```python
from build123d import *

# Parameters (mm, degrees)
F0_W                 = 20
F0_H                 = 40
F0_R                 = 3
F0_H_2               = 20
F0_R_2               = 5
F0_W_2               = 40
F1_DEPTH             = 3
F0_W_3               = 3
F0_H_3               = 3
F2_DEPTH             = 23
F3_DEPTH             = 63
F4_R                 = 3
F4_R_2               = 5
F6_DEPTH             = 25
F5_R                 = 3
F5_R_2               = 5
F7_DEPTH             = 25
F8_DEPTH             = 23
F9_D                 = 6
F9_DEPTH             = 23
F9_CBORE_D           = 10
F9_CBORE_DEPTH       = 21
F9_TIP               = 1.8025818571
F9_ON_F5_D           = 6
F9_ON_F5_DEPTH       = 23
F9_ON_F5_CBORE_D     = 10
F9_ON_F5_CBORE_DEPTH = 21
F9_ON_F5_TIP         = 1.8025818571
F9_ON_F4_D           = 6
F9_ON_F4_DEPTH       = 23
F9_ON_F4_CBORE_D     = 10
F9_ON_F4_CBORE_DEPTH = 21
F9_ON_F4_TIP         = 1.8025818571


# Not quite as in the source:
# - a feature of the source that left no trace in its solid (it failed there, or was rolled back) is left out


with BuildPart() as f1:
    # F0 (on Front) → F1 (new body)
    with BuildSketch(Plane.XZ):
        with Locations((-10, 20)):
            Rectangle(F0_W, F0_H)
        with Locations((-10, 7.5)):
            Circle(F0_R, mode=Mode.SUBTRACT)
        with Locations((-10, 32.5)):
            Circle(F0_R, mode=Mode.SUBTRACT)
        with Locations((-10, 50)):
            Rectangle(F0_W, F0_H_2)
        with Locations((-10, 50)):
            Circle(F0_R_2, mode=Mode.SUBTRACT)
        with Locations((20, 50)):
            Rectangle(F0_W_2, F0_H_2)
        with Locations((7.5, 50)):
            Circle(F0_R, mode=Mode.SUBTRACT)
        with Locations((32.5, 50)):
            Circle(F0_R, mode=Mode.SUBTRACT)
    extrude(amount=-F1_DEPTH)

    # F0 (on Front) → F2 (join)
    with BuildSketch(Plane.XZ):
        with Locations((-21.5, 20)):
            Rectangle(F0_W_3, F0_H)
        with Locations((20, 61.5)):
            Rectangle(F0_W_2, F0_H_3)
    extrude(amount=-F2_DEPTH)

    # F0 (on Front) → F3 (join)
    with BuildSketch(Plane.XZ):
        Polygon((-20, 60), (0, 60), (0, 63), (-23, 63), (-23, 60), align=None)
        with Locations((-21.5, 50)):
            Rectangle(F0_W_3, F0_H_2)
    extrude(amount=-F3_DEPTH)

    # F4 (on face) → F6 (cut)
    with BuildSketch(Plane.XY.offset(63)):
        with Locations((-10, 55.5)):
            Circle(F4_R)
        with Locations((-10, 30.5)):
            Circle(F4_R)
        with Locations((-10, 13)):
            Circle(F4_R_2)
        with Locations((7.5, 13)):
            Circle(F4_R)
        with Locations((32.5, 13)):
            Circle(F4_R)
    extrude(amount=-F6_DEPTH, mode=Mode.SUBTRACT)

    # F5 (on face) → F7 (cut)
    with BuildSketch(Plane(origin=(-23, 0, 0), x_dir=(0, -1, 0), z_dir=(-1, 0, 0))):
        with Locations((-55.5, 50)):
            Circle(F5_R)
        with Locations((-30.5, 50)):
            Circle(F5_R)
        with Locations((-13, 50)):
            Circle(F5_R_2)
        with Locations((-13, 7.5)):
            Circle(F5_R)
        with Locations((-13, 32.5)):
            Circle(F5_R)
    extrude(amount=-F7_DEPTH, mode=Mode.SUBTRACT)

    # F0 (on Front) → F8 (join)
    with BuildSketch(Plane.XZ):
        with Locations((-10, 50)):
            Rectangle(F0_W, F0_H_2)
        with Locations((-10, 50)):
            Circle(F0_R_2, mode=Mode.SUBTRACT)
        Polygon((-20, 60), (0, 60), (0, 63), (-23, 63), (-23, 60), align=None)
        with Locations((-21.5, 50)):
            Rectangle(F0_W_3, F0_H_2)
        with Locations((-10, 50)):
            Circle(F0_R_2)
    extrude(amount=-F8_DEPTH)

    # F9
    with Locations(Plane.XZ):
        with Locations((-10, 50)):
            CounterBoreHole(F9_D / 2, F9_CBORE_D / 2, F9_CBORE_DEPTH, depth=F9_DEPTH)
            with Locations((0, 0, -(F9_DEPTH + F9_TIP / 2))):  # 118° drill point
                Cone(0, F9_D / 2, F9_TIP, mode=Mode.SUBTRACT)

    # F9 on F5
    with Locations(Plane(origin=(-23, 0, 0), x_dir=(0, -1, 0), z_dir=(-1, 0, 0))):
        with Locations((-13, 50)):
            CounterBoreHole(F9_ON_F5_D / 2, F9_ON_F5_CBORE_D / 2, F9_ON_F5_CBORE_DEPTH, depth=F9_ON_F5_DEPTH)
            with Locations((0, 0, -(F9_ON_F5_DEPTH + F9_ON_F5_TIP / 2))):  # 118° drill point
                Cone(0, F9_ON_F5_D / 2, F9_ON_F5_TIP, mode=Mode.SUBTRACT)

    # F9 on F4
    with Locations(Plane.XY.offset(63)):
        with Locations((-10, 13)):
            CounterBoreHole(F9_ON_F4_D / 2, F9_ON_F4_CBORE_D / 2, F9_ON_F4_CBORE_DEPTH, depth=F9_ON_F4_DEPTH)
            with Locations((0, 0, -(F9_ON_F4_DEPTH + F9_ON_F4_TIP / 2))):  # 118° drill point
                Cone(0, F9_ON_F4_D / 2, F9_ON_F4_TIP, mode=Mode.SUBTRACT)


solid = f1.part
```
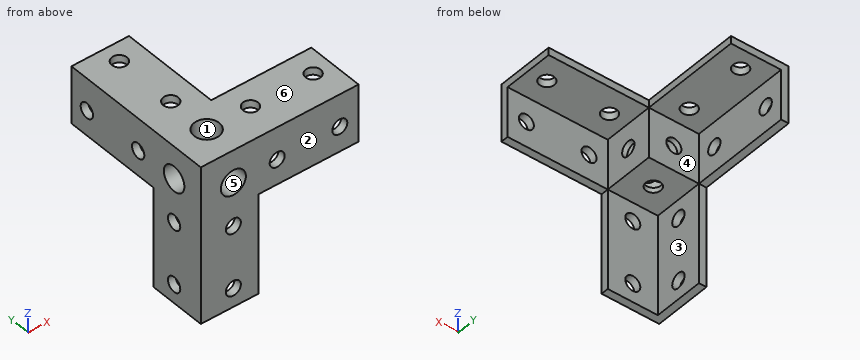
Work out the finished part from the listing and answer in its coordinate system (mm). Face numbers are marked on the shaded views. A direction names the side the tool comes from. Round coordinates to 2 decimals unless told otherwise and drop trailing zeros. Loops run counter-clockwise (first coordinate to the right, second up) from the corner with the lowest first, then second, coordinate; pieces in that order, holes last. Notation, with made-up numbers: M 70,-37.5 L 111,-37.5 A15 cw 111,-20.5 Z; hole C 87.5,24 d6. An arc over 180 degrees is marked long. One line per question, with ' | ' between items.
Q1. Find section C-C, the plane y = 5.5. Give the vertices of the cut face in (x, z).
Conclusion:
outline: M -23,0 L -20,0 L -20,40 L 0,40 L 0,60 L 40,60 L 40,63 L -23,63 Z; hole C -10,50 d10
Q2. Find section A-A, the plane x = 32.5. Give the vertices of the cut face in (y, z), then the cut area to 3 significant figures.
Conclusion:
outline: M 0,40 L 3,40 L 3,47 L 0,47 Z; M 0,53 L 3,53 L 3,60 L 10,60 L 10,63 L 0,63 Z; M 16,60 L 23,60 L 23,63 L 16,63 Z | area: 93.0 mm2
Q3. A tool of negligible diameter and unlimited length cuts with its end or side. For the marked faces 4, 5 and 6, from which of +Z, -Z, +X, -X, +Y, -Y can it reach the whole face along a straight path? Write none if from no direction.
Conclusion:
face 4: -Z, +X, +Y | face 5: -Y | face 6: +Z, +X, -X, +Y, -Y
Q4. Find section D-D, the plane z = 25.5. Give the vertices of the cut face in (x, y).
Conclusion:
outline: M -23,0 L 0,0 L 0,3 L -20,3 L -20,23 L -23,23 Z
Q5. Find section B-B, the plane y = 30.5. Give the vertices of the cut face in (x, z), then the cut area to 3 significant figures.
Conclusion:
outline: M -23,40 L -20,40 L -20,47 L -23,47 Z; M -23,53 L -20,53 L -20,60 L -13,60 L -13,63 L -23,63 Z; M -7,60 L 0,60 L 0,63 L -7,63 Z | area: 93.0 mm2
Q6. Each of these flat-tipped pins is pushed along its axis until it touches: pin 1 Ø10 at (y, z) = (11, 53) entering from +X; pin 2 Ø11 at (x, y) = (-12, 14.5) entering from +Z; pin 3 Ø8 at (x, y) = (7.5, 13) entering from -Z; pin 4 Ø7 at (y, z) = (13, 32.5) entering from +X. Where does it stop, or does it pass through?
Conclusion:
pin 1: stops at x = 0 | pin 2: stops at z = 63 | pin 3: stops at z = 60 | pin 4: stops at x = -20
Q7. Consider line 1 along Y through (x, z) = (-10, 61); line 2 along Z through (x, y) = (7.5, 1.95); line 3 along X through (y, z) = (13, 43). Determine where each line is inside the solid, lowest interval first. Write a range as from..to.
Conclusion:
line 1: y = 0..8, 18..27.5, 33.5..52.5, 58.5..63 | line 2: z = 40..47, 53..63 | line 3: x = -23..-15, -5..0
Q8. The mould has two halves that part along Y. Classify the marked faces 1, 2 and 3: +Y half, -Y half, draft (parallel to the pull), parting line (faces both ways), or undercut.
Conclusion:
face 1: undercut | face 2: -Y half | face 3: draft
